Source: three-view drawing plus pictorial views. Frame: mm from the lowest corner of the part. A direction names the side the tool comes from. Coordinates: 2 decimals unless noted, no trailing zeros. Loops run counter-clockwise (first coordinate to the right, second up) from the corner with the lowest first, then second, coordinate; pieces in that order, holes last. Notation, with made-up numbers: M 37.5,19 L 62.5,19 A33 ccw 62.5,58 Z; hole C -6.5,-8 d4. An arc over 180 degrees is marked long. Use a Markdown table: item, result. Add a question column.
1. Set-up query: the marked faces 5 and 6. Return all of +Z, -Z, +X, -X, +Y, -Y with unobstructed straight access to the full face (end or side cutting, diameter ignored); none if empty.
2. Section B-B on z = 1.3. State how many separate pieces and enclosed holes the cut face has.
3. Section C-C on x = 17.5. Output: boundary loops of the cut face in (y, z).
4. Draft query along Y for the marked faces 1, 2, 3 and 4. Return one class per face: +Y half, -Y half, draft (parallel to the pull), parting line (faces both ways), or undercut.
5. Line query: L1, parallel to Y at x = 30, z = 2.15; L2, parallel to X at y = 10.5, z = 5.75 (1 decimal); L3, parallel to X at y = 9.25, z = 1.6. Output: solid intervals per line, ascending. Write a range as [from, to].
6. Pin query (flat end, axial travel): pin 1 (3.5 mm diameter, centred on x = 5, y = 10, fed in from +Z) (1 decimal). Return the tip coordinate at first contact, or that it passes through.
7. Section A-A on x = 30. Output: boundary loops of the cut face in (y, z).
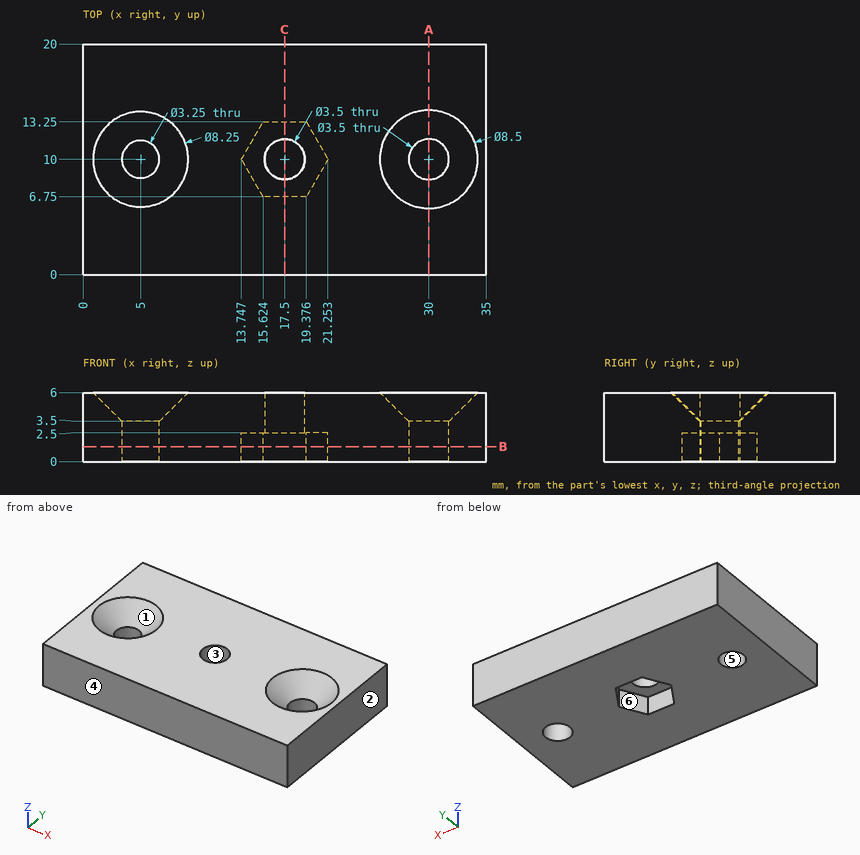
Answers below:
| question | item | result |
|---|---|---|
| 1 | face 5 | +Z, -Z |
| 1 | face 6 | -Z |
| 2 | separate pieces | 1 |
| 2 | enclosed holes | 3 |
| 3 | outline | M 0,0 L 6.75,0 L 6.75,2.5 L 8.25,2.5 L 8.25,6 L 0,6 Z; M 11.75,2.5 L 13.25,2.5 L 13.25,0 L 20,0 L 20,6 L 11.75,6 Z |
| 4 | face 1 | undercut |
| 4 | face 2 | draft |
| 4 | face 3 | undercut |
| 4 | face 4 | -Y half |
| 5 | L1 | y = [0, 8.25], [11.75, 20] |
| 5 | L2 | x = [0, 1.2], [8.8, 15.8], [19.2, 26], [34, 35] |
| 5 | L3 | x = [0, 3.56], [6.44, 14.18], [20.82, 28.42], [31.58, 35] |
| 6 | pin 1 | stops at z = 3.6 |
| 7 | outline | M 0,0 L 8.25,0 L 8.25,3.5 L 5.75,6 L 0,6 Z; M 11.75,0 L 20,0 L 20,6 L 14.25,6 L 11.75,3.5 Z |
